Source: CAD feature listing. Evaluate the final solid. Frame: model axes, mm. Face numbers are marked on the shaded views. A direction names the side the tool comes from. Give positions to 0.01 mm unless a question says otherwise; leave off trailing zeros. Loops run counter-clockwise (first coordinate to the right, second up) from the corner with the lowest first, then second, coordinate; pieces in that order, holes last. Notation, with made-up numbers: (42, -4) -> (84, -4) arc R6 ccw to (84, 6) -> close; hole circle Ø10 at (85, -26). An arc over 180 degrees is marked (long way). Answer as a JSON object with one key per item and string values. Group by question number.
from build123d import *

# Parameters (mm, degrees)
SKETCH_1_W             = 30
SKETCH_1_H             = 30
SM_BASE_FLANGE_1_DEPTH = 0.5
SM_EDGE_FLANGE_1_DEPTH = 30
HOLE_WIZARD_M6_1_D     = 5
HOLE_WIZARD_M6_1_DEPTH = 15
HOLE_WIZARD_M6_1_TIP   = 1.502151548


# Sheet-metal steps are written as plain solids
with BuildPart() as part:
    # Sketch 1 → 基体-法兰1 (new body)
    with BuildSketch(Plane.XY):
        Rectangle(SKETCH_1_W, SKETCH_1_H)
    extrude(amount=-SM_BASE_FLANGE_1_DEPTH)

    # 边线-法兰1 section (across the edge) → 边线-法兰1 (add)
    with BuildSketch(Plane(origin=(-15.5, 15, 0), x_dir=(1, 0, 0), z_dir=(0, -1, 0))):
        with BuildLine():
            Line((-0.5, 0.5), (-0.5, 26.5))
            Line((-0.5, 26.5), (0, 26.5))
            Line((0, 26.5), (0, 0.5))
            ThreePointArc((0, 0.5), (0.146446609, 0.146446609), (0.5, 0))
            Line((0.5, 0), (0.5, -0.5))
            ThreePointArc((0.5, -0.5), (-0.207106781, -0.207106781), (-0.5, 0.5))
        make_face()
    extrude(amount=SM_EDGE_FLANGE_1_DEPTH)

    # M6 螺纹孔的螺纹孔钻头1
    with Locations(Plane(origin=(-15.5, 0, 16.512507822), x_dir=(0, 0, 1), z_dir=(1, 0, 0))):
        with Locations((0, 0)):
            Hole(HOLE_WIZARD_M6_1_D / 2, depth=HOLE_WIZARD_M6_1_DEPTH)
            with Locations((0, 0, -(HOLE_WIZARD_M6_1_DEPTH + HOLE_WIZARD_M6_1_TIP / 2))):  # 118° drill point
                Cone(0, HOLE_WIZARD_M6_1_D / 2, HOLE_WIZARD_M6_1_TIP, mode=Mode.SUBTRACT)


solid = part.part
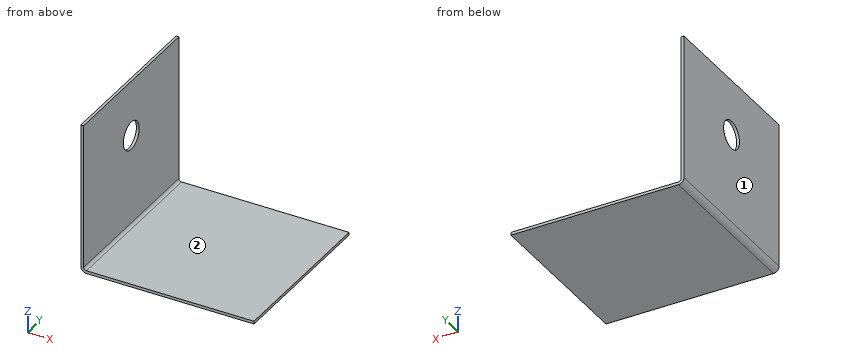
(1) Section query D-D on x = -1. Return the cut outline in (y, z), plus the area to 3 significant figures.
(2) First-contact query: pin 1 (9 mm diameter, centred on x = -3, y = 0, fed in from +Z); pin 2 (5 mm diameter, centred on x = -12, z = 6.5, fed in from +Y) (3 decimals); pin 3 (3 mm diameter, centred on y = -0.5, z = 2.5, fed in from +X). Flat tips, straight axial feed; report the tip coordinate or a pass-through.
(3) Section query C-C on z = 24.25. Return the cut outline in (x, y), plus the area to 3 significant figures.
(4) Material intervals for line 1 (X direction, y = 6.25, z = 15.25); line 2 (Z direction, x = 6.5, y = -9.5), sorted ascending. Write a range as from..to.
(5) Access query for the marked faces 1 and 2. Directions: +Z, -Z, +X, -X, +Y, -Y. A direction counts if a zero-diameter tool reaches every point of the face in a straight line with its end or side. Return the directions, or none.
(6) Section query B-B on y = -9.75. Return the cut outline in (x, z).
(7) Section query A-A on y = 0. Return the cut outline in (x, z).
Result:
{
 "1": {"outline": "(-15, -0.5) -> (15, -0.5) -> (15, 0) -> (-15, 0) -> close", "area": "15.0 mm²"},
 "2": {"pin 1": "z = 0", "pin 2": "through", "pin 3": "x = -15.5"},
 "3": {"outline": "(-16, -15) -> (-15.5, -15) -> (-15.5, 15) -> (-16, 15) -> close", "area": "15.0 mm²"},
 "4": {"line 1": "-16..-15.5", "line 2": "-0.5..0"},
 "5": {"face 1": "+Z, -Z, -X, +Y, -Y", "face 2": "+Z, +X, +Y, -Y"},
 "6": {"outline": "(-16, 0.5) arc R1 ccw to (-15, -0.5) -> (15, -0.5) -> (15, 0) -> (-15, 0) arc R0.5 cw to (-15.5, 0.5) -> (-15.5, 26.5) -> (-16, 26.5) -> close"},
 "7": {"outline": "(-16, 0.5) arc R1 ccw to (-15, -0.5) -> (15, -0.5) -> (15, 0) -> (-15, 0) arc R0.5 cw to (-15.5, 0.5) -> (-15.5, 14.01) -> (-16, 14.01) -> close; (-16, 19.01) -> (-15.5, 19.01) -> (-15.5, 26.5) -> (-16, 26.5) -> close"}
}
